Work out the finished part from the listing and answer in its coordinate system (mm). A direction names the side the tool comes from. Give positions to 0.01 mm unless a question says otherwise; leave off trailing zeros. Write each loop counter-clockwise with the first axis right and the second up, starting at its lowest first coordinate (ties: lowest second). Pieces come first, ordered by that corner, then holes. Notation, with made-up numbers: (-29.5, 85.5) -> (3.5, 85.5) arc R21 ccw to (3.5, 122.5) -> close; hole circle Ø10 at (33, -0.5). An arc over 180 degrees is marked (long way). Write item = value, one per line. Start each with the question number.
Autodesk Inventor part; units mm, degrees
ref_plane "Work Plane1" through (0, 20, 0) normal (0, 1, 0) x (1, 0, 0)
ref_plane "YZ Plane" through (0, 0, 0) normal (1, 0, 0) x (0, 1, 0)
ref_plane "XZ Plane" through (0, 0, 0) normal (0, 1, 0) x (-1, 0, 0)
sketch "Sketch1" plane through (0, 0, 0) normal (0, 1, 0) x (-1, 0, 0)
  line L0 (0, 0) -> (74.5, 0)
  line L1 (74.5, 0) -> (74.5, -40)
  line L2 (74.5, -40) -> (0, -40)
  line L3 (0, -40) -> (0, 0)
  line L4 (74.5, -40) -> (77.5, -40)
  line L5 (77.5, -40) -> (77.5, 0)
  line L6 (77.5, 0) -> (74.5, 0)
  line L7 (74.5, 0) -> (74.5, -40)
  line L8 (0, -40) -> (-3, -40)
  line L9 (-3, -40) -> (-3, 0)
  line L10 (-3, 0) -> (0, 0)
  line L11 (0, 0) -> (0, -40)
  line L12 (-3, 0) -> (77.5, 0)
  line L13 (77.5, 0) -> (77.5, 5)
  line L14 (77.5, 5) -> (-3, 5)
  line L15 (-3, 5) -> (-3, 0)
  dimension "d0" = 74.5
  dimension "d1" = 40
  dimension "d2" = 3
  dimension "d3" = 3
  dimension "d4" = 40
  dimension "d5" = 80.5
  dimension "d6" = 5
extrude "Extrusion1" add sketch "Sketch1" along normal blind 40 contours L10 L15 L14 L13 L6 L0 | L3 L8 L9 L10 | L6 L5 L4 L1
sketch "Sketch3" plane through (0, 0, 0) normal (0, 0, -1) x (-1, 0, 0)
  line L0 (0, 0) -> (14.225, 0)
  line L1 (0, 0) -> (74.5, 0)
  line L2 (14.225, 0) -> (14.225, 8)
  circle A0 centre (14.225, 8) radius 3
  line L3 (37.25, 0) -> (37.25, 20.4526)
  line L4 (74.5, 0) -> (74.5, 40)
  line L5 (74.5, 0) -> (74.5, 8)
  line L6 (74.5, 8) -> (62.265, 8)
  line L7 (74.5, 8) -> (86.735, 8) construction
  circle A1 centre (62.265, 8) radius 3
  dimension "d9" = 14.225
  dimension "d10" = 8
  dimension "d11" = 6
  dimension "d12" = 8
  dimension "d13" = 12.235
  dimension "d14" = 180
  dimension "d15" = 6
extrude "Extrusion2" add sketch "Sketch3" along normal blind 4
chamfer "Chamfer1" distance 1 angle 45 2 edges at (-11.225, 8, -4) (-59.265, 8, -4)
sketch "Sketch4" plane through (0, 40, 0) normal (0, 1, 0) x (1, 0, 0)
  line L0 (3, -5) -> (3, 40)
  line L1 (-77.5, 40) -> (-77.5, -5)
  line L2 (3, 40) -> (-77.5, 40)
  line L3 (-77.5, 40) -> (-77.5, 39)
  line L4 (-77.5, 39) -> (3, 39)
  line L5 (3, 39) -> (3, 40)
  point P0 (0, 0)
  dimension "d21" = 1
extrude "Extrusion3" cut sketch "Sketch4" against normal blind 40
ref_plane "Work Plane1" through (0, 20, 0) normal (0, 1, 0) x (1, 0, 0)
sketch "Sketch6" plane through (0, 20, 0) normal (0, 1, 0) x (1, 0, 0)
  line L0 (0, 39) -> (3, 39)
  line L1 (3, 39) -> (13, 39)
  line L2 (13, 39) -> (13, 24)
  line L3 (13, 24) -> (3, 24)
  line L4 (3, 24) -> (3, 39)
  line L5 (0, 0) -> (-74.5, 0)
  line L6 (-37.25, 0) -> (-37.25, 6.791)
  line L7 (-74.5, 39) -> (-77.5, 39)
  line L8 (-77.5, 39) -> (-87.5, 39)
  line L9 (-87.5, 39) -> (-87.5, 24)
  line L10 (-87.5, 24) -> (-77.5, 24)
  line L11 (-77.5, 24) -> (-77.5, 39)
  dimension "d24" = 10
  dimension "d25" = 15
extrude "Extrusion4" add sketch "Sketch6" along normal mid plane 14
chamfer "Chamfer2" distance 10 angle 45 1 edges at (-87.5, 20, -24)
chamfer "Chamfer3" distance 10 angle 45 1 edges at (13, 20, -24)
sketch "Sketch7" plane through (-74.5, 40, -39) normal (0, 0, -1) x (-1, 0, 0)
  line L0 (13, -27) -> (13, -13)
  line L1 (3, -13) -> (13, -13)
  line L2 (13, -13) -> (3, -13)
  line L3 (13, -13) -> (13, -27)
  line L4 (13, -20) -> (8, -20)
  circle A0 centre (8, -20) radius 1.375
  line L5 (-74.5, 0) -> (0, 0)
  line L6 (-37.25, 0) -> (-37.25, -5.3996)
  circle A1 centre (-82.5, -20) radius 1.375
  point P0 (-74.5, -40)
  dimension "d34" = 5
  dimension "d35" = 2.75
extrude "Extrusion5" cut sketch "Sketch7" against normal blind 14
sketch "Sketch9" plane through (0, 40, 0) normal (0, 1, 0) x (1, 0, 0)
  line L0 (-77.5, 39) -> (-77.5, -5)
  line L1 (13, 39) -> (3, 39)
  line L2 (-77.5, -5) -> (3, -5)
  line L3 (3, 39) -> (-77.5, 39)
  line L4 (-77.5, 39) -> (-77.5, -5)
  line L5 (-37.25, 39) -> (-37.25, 40)
  line L6 (-37.25, 39) -> (-36.25, 39) construction
  circle A0 centre (-37.25, 40) radius 62
  circle A1 centre (-37.25, 40) radius 55
  line L7 (-37.25, 40) -> (-42.25, 40)
  line L8 (-42.25, 40) -> (-32.25, 40)
  line L9 (-32.25, 40) -> (-32.25, -25)
  line L10 (-32.25, -25) -> (-42.25, -25)
  line L11 (-42.25, -25) -> (-42.25, 40)
  line L12 (-37.25, 39) -> (-127.25, 39)
  line L13 (-37.25, 39) -> (52.75, 39) construction
  line L14 (-127.25, 39) -> (47.7384, 39)
  line L15 (-77.5, 39) -> (-77.5, 24)
  line L16 (-77.5, 39) -> (-93.5, 39)
  line L17 (-93.5, 39) -> (-93.5, 36)
  line L18 (-92.1044, 36) -> (-77.5, 36)
  line L19 (-77.5, 36) -> (-77.5, 39)
  line L20 (3, -5) -> (3, 39)
  line L21 (3, 39) -> (19, 39)
  line L22 (19, 39) -> (19, 36)
  line L23 (17.6044, 36) -> (3, 36)
  line L24 (3, 36) -> (3, 39)
  line L25 (3, 39) -> (19, 39)
  line L26 (19, 39) -> (19, 36)
  line L27 (17.6044, 36) -> (3, 36)
  line L28 (3, 36) -> (3, 39)
  line L29 (3, -5) -> (3, 2.5175)
  line L30 (3, 36) -> (3, 39)
  point P0 (0, 0)
  point P1 (3, 2.5175)
  point P2 (-5.6272, -5)
  point P3 (-32.25, -14.7723)
  point P4 (-32.25, -5)
  point P5 (-42.25, -5)
  point P6 (-42.25, -14.7723)
  point P7 (-68.8728, -5)
  point P8 (-77.5, 2.5175)
  point P9 (-99.2419, 39)
  point P10 (24.7419, 39)
  dimension "d38" = 1
  dimension "d39" = 90
  dimension "d40" = 124
  dimension "d41" = 110
  dimension "d42" = 5
  dimension "d43" = 10
  dimension "d44" = 65
  dimension "d45" = 90
  dimension "d46" = 180
  dimension "d47" = 16
  dimension "d48" = 3
  dimension "d49" = 16
  dimension "d50" = 3
extrude "Extrusion6" add sketch "Sketch9" against normal blind 13 contours L0 L18 A1 L12 | A1 L0 L2 L11 A0 L12 | L2 L9 A1 L11 | A1 L9 A0 L11 | L14 A0 L9 A1 L2 L20 | A1 L23 L20 L1 L14
sketch "Sketch10" plane through (0, 40, 0) normal (0, 1, 0) x (1, 0, 0)
  arc A0 (-99.2419, 39) -> (24.7419, 39) centre (-37.25, 40) ccw
  line L0 (-37.25, -22) -> (-37.25, -10)
  circle A1 centre (-37.25, -10) radius 1.375
  point P0 (0, 0)
  dimension "d53" = 12
  dimension "d54" = 2.75
extrude "Extrusion7" cut sketch "Sketch10" against normal blind 13
sketch "Sketch11" plane through (0, 27, 0) normal (0, -1, 0) x (1, 0, 0)
  circle A0 centre (-37.25, 10) radius 1.375
  line L0 (-37.25, 10) -> (-37.25, 12)
  line L1 (-37.25, 12) -> (-37.25, 8)
  arc A1 (-38.374, 9.208) -> (-36.126, 9.208) centre (-37.25, 8) ccw
  arc A2 (-36.126, 10.792) -> (-38.374, 10.792) centre (-37.25, 12) ccw
  line L2 (-38.9, 12) -> (-38.9, 8)
  line L3 (-35.6, 8) -> (-35.6, 12)
  point P0 (0, 0)
  point P1 (-38.625, 10.25)
  point P2 (-35.875, 10.25)
  dimension "d57" = 2
  dimension "d58" = 4
  dimension "d59" = 3.3
  dimension "d60" = 3.3
extrude "Extrusion8" cut sketch "Sketch11" against normal blind 13 contours A0 A2 | A1 A0
sketch "Sketch12" plane through (0, 27, 0) normal (0, -1, 0) x (1, 0, 0)
  point P0 (0, 0)
sketch "Sketch13" plane through (0, 40, 0) normal (0, 1, 0) x (1, 0, 0)
  arc A0 (-99.2419, 39) -> (24.7419, 39) centre (-37.25, 40) ccw
  circle A1 centre (-37.25, 40) radius 62.25
  line L0 (-42.25, -14.7723) -> (-42.25, -5)
  circle A2 centre (-37.25, 40) radius 55
  line L1 (-32.25, -5) -> (-42.25, -5)
  line L2 (-32.25, -14.7723) -> (-32.25, -5)
  line L3 (-42.25, -5) -> (-32.25, -5)
  line L4 (-32.25, -5) -> (-32.25, -14.7723)
  line L5 (-42.25, -14.7723) -> (-42.25, -5)
  point P0 (0, 0)
extrude "Extrusion9" cut sketch "Sketch13" against normal blind 7 contours L0 L1 L2 A2 picked at (-36.6938, -8.3249)
sketch "Sketch14" plane through (0, 27, 0) normal (0, -1, 0) x (1, 0, 0)
  arc A0 (-36.126, 10.792) -> (-38.374, 10.792) centre (-37.25, 12) ccw
  arc A1 (-35.6, 12) -> (-38.9, 12) centre (-37.25, 12) ccw
  arc A2 (-38.374, 9.208) -> (-36.126, 9.208) centre (-37.25, 8) ccw
  arc A3 (-38.9, 8) -> (-35.6, 8) centre (-37.25, 8) ccw
  line L0 (-35.6, 12) -> (-35.6, 8)
  line L1 (-38.9, 8) -> (-38.9, 12)
  point P0 (0, 0)
extrude "Extrusion10" cut sketch "Sketch14" against normal blind 10
sketch "Sketch15" plane through (0, 27, 0) normal (0, -1, 0) x (1, 0, 0)
  arc A0 (-5.6272, 5) -> (-68.8728, 5) centre (-37.25, -40) ccw
  line L0 (-42.25, 14.7723) -> (-42.25, 5)
  circle A1 centre (-37.25, -40) radius 55
  circle A2 centre (-37.25, -40) radius 62
  circle A3 centre (-37.25, -40) radius 59
  line L1 (-37.25, -40) -> (-35.25, -40)
  line L2 (-35.25, -40) -> (-39.25, -40)
  line L3 (-39.25, -40) -> (-39.25, 33.7225)
  line L4 (-39.25, 33.7225) -> (-35.25, 33.7225)
  line L5 (-35.25, 33.7225) -> (-35.25, -40)
  line L6 (-39.25, 33.7225) -> (-35.25, 33.7225)
  line L7 (-35.25, 33.7225) -> (-35.25, -40)
  line L8 (-35.25, -40) -> (-39.25, -40)
  line L9 (-39.25, -40) -> (-39.25, 33.7225)
  point P0 (0, 0)
  point P1 (-39.25, 21.9677)
  point P2 (-39.25, 18.9661)
  point P3 (-35.25, 18.9661)
  point P4 (-35.25, 21.9677)
  dimension "d67" = 118
  dimension "d68" = 2
  dimension "d69" = 4
extrude "Extrusion11" cut sketch "Sketch15" against normal blind 8 contours L3 A2 L5 A3 picked at (-35.6944, 19.9767)
chamfer "Chamfer4" distance 2 angle 45 2 edges at (-35.25, 27, 20.4669) (-39.25, 27, 20.4669)
sketch "Sketch16" plane through (0, 40, 0) normal (0, 1, 0) x (1, 0, 0)
  arc A0 (3, 2.5175) -> (17.6044, 36) centre (-37.25, 40) ccw
  circle A1 centre (-37.25, 40) radius 59
  circle A2 centre (-37.25, 40) radius 62
  line L0 (24.7419, 39) -> (0, 39)
  line L1 (24.7419, 39) -> (21.7415, 39)
  arc A3 (-99.2419, 39) -> (24.7419, 39) centre (-37.25, 40) ccw
  line L2 (-99.2419, 39) -> (-96.2415, 39)
  line L3 (-74.5, 39) -> (-99.2419, 39)
  point P0 (0, 0)
  dimension "d75" = 118
extrude "Extrusion12" add sketch "Sketch16" along normal blind 2 contours A1 L0 A2 L2 picked at (-37.25, -19.8358)
sketch "Sketch17" plane through (0, 42, 0) normal (0, 1, 0) x (1, 0, 0)
  arc A0 (-68.8728, -5) -> (-5.6272, -5) centre (-37.25, 40) ccw
  circle A1 centre (-37.25, 40) radius 59
  circle A2 centre (-37.25, 40) radius 68
  line L0 (3, 39) -> (13, 39)
  line L1 (13, 39) -> (38.5571, 39)
  line L2 (13, 39) -> (24.7419, 39)
  line L3 (38.5571, 39) -> (-112.8273, 39)
  point P0 (0, 0)
  point P1 (-96.2415, 39)
  point P2 (-105.2426, 39)
  point P3 (30.7426, 39)
  point P4 (21.7415, 39)
  dimension "d78" = 136
extrude "Extrusion13" add sketch "Sketch17" along normal blind 2 contours A1 L1 A2 L3 picked at (-35.4549, -24.766)
chamfer "Chamfer5" distance 4 angle 45 2 edges at (3, 13.5, 5) (-77.5, 13.5, 5)
properties part number "gripper_mount_female"
(1) For faces 1 (the flat face through (-48, 42, 22)), 2 (the flat face through (7, 27, -31)), 3 (the flat face through (-33, 40, 1)), 4 (the cylindrical face through (-65.126, 7.099, -1.479)), determine the directions among +Z, -Z, +X, -X, +Y, -Y from which every point of the face is accessible in a straight line to the end or side of a thin tool.
(2) A cutting plane is placed at B-B, the plane z = -32.5. State how many separate pieces and enclosed holes the cut face has, then the cut area to 3 significant figures.
(3) A cutting plane is placed at A-A, the plane x = -37.25. Write down the section's boundary in (y, z).
(4) Find the intervals of material crossed by line 1 along X through (y, z) = (20, -35) (3 decimals); line 2 along X through (y, z) = (9.5, -22.5); line 3 along X through (y, z) = (35, -20.5), in increasing order.
(5) Determine the mould class of faces 5 (the cylindrical face through (-11.228, 7.868, -1.479)), 6 (the flat face through (10, 34, -36)), 7 (the flat face through (1, 13, 3)) for opening direction Z: pulls with the +Z half, pulls with the -Z half, needs draft (parallel to the pull), parting line crosses it, or undercut.
(6) Each of these flat-tipped pins is pushed along its axis until it touches: pin 1 (20 mm diameter, centred on y = 29.5, z = -19.5, fed in from -X); pin 2 (2.5 mm diameter, centred on y = 19.5, z = -36, fed in from +X); pin 3 (2 mm diameter, centred on y = 30.5, z = 9.5, fed in from -X). Where does it stop, or does it pass through?
(7) A cutting plane is placed at C-C, the plane z = -6. Write down the section's boundary in (x, y).
Results list:
q1.face_1 = +Z, -Y
q1.face_2 = +Y
q1.face_3 = -Z, +Y
q1.face_4 = -Z
q2.separate_pieces = 4
q2.enclosed_holes = 2
q2.area = 698 mm²
q3.outline = (0, 0) -> (40, 0) -> (40, 5) -> (33, 5) -> (33, 6.35) -> (27, 6.35) -> (27, 5) -> (0, 5) -> close; (27, 13.65) -> (33, 13.65) -> (33, 15) -> (40, 15) -> (40, 19) -> (44, 19) -> (44, 28) -> (42, 28) -> (42, 22) -> (35, 22) -> (35, 19) -> (27, 19) -> close
q4.line_1 = -87.5 to -83.875, -81.125 to -74.5, 0 to 6.625, 9.375 to 13
q4.line_2 = -77.5 to -74.5, 0 to 3
q4.line_3 = -96.1 to -88.68, -77.5 to -74.5, 0 to 3, 14.18 to 21.6
q5.face_5 = needs draft
q5.face_6 = undercut
q5.face_7 = pulls with the +Z half
q6.pin_1 = -98.35
q6.pin_2 = 13
q6.pin_3 = -75.87
q7.outline = (-96.14, 42) -> (-89.1, 42) -> (-89.1, 27) -> (-80.48, 27) -> (-80.48, 40) -> (-85.47, 40) -> (-85.47, 44) -> (-96.14, 44) -> close; (-77.5, 0) -> (-74.5, 0) -> (-74.5, 40) -> (-77.5, 40) -> close; (0, 0) -> (3, 0) -> (3, 40) -> (0, 40) -> close; (5.98, 27) -> (14.6, 27) -> (14.6, 42) -> (21.64, 42) -> (21.64, 44) -> (10.97, 44) -> (10.97, 40) -> (5.98, 40) -> close
